Read the model definition and answer for the solid it produces. Units are mm, in the model's axes. Coordinates: 2 decimals unless noted, no trailing zeros. Write each loop counter-clockwise with the first axis right and the second up, starting at its lowest first coordinate (ties: lowest second). Pieces come first, ordered by that corner, then holes. Notation, with made-up numbers: (-23, 60.25) - (-10, 60.25) arc R23 ccw to (-10, 97.25) - close; hole circle Ø4 at (71, 35.5). An arc over 180 degrees is marked (long way). Use a Markdown table: item, result.
from build123d import *

# Parameters (mm, degrees)
ESBO_O1_W                = 45
ESBO_O1_H                = 27
RESSALTO_EXTRUS_O1_DEPTH = 1.7
RESSALTO_EXTRUS_O2_DEPTH = 1
ESBO_O3_R                = 1
CORTE_EXTRUS_O1_DEPTH    = 2.7


with BuildPart() as part:
    # Esboço1 → Ressalto-extrusão1 (new body)
    with BuildSketch(Plane(origin=(0, 0, 0), x_dir=(1, 0, 0), z_dir=(0, 1, 0))):
        with Locations((22.5, 13.5)):
            Rectangle(ESBO_O1_W, ESBO_O1_H)
    extrude(amount=RESSALTO_EXTRUS_O1_DEPTH)

    # Esboço2 → Ressalto-extrusão2 (add)
    with BuildSketch(Plane.XZ):
        Polygon((3, -22.5), (5, -24.5), (40, -24.5), (42, -22.5), (42, -4.5), (40, -2.5), (5, -2.5), (3, -4.5), align=None)
    extrude(amount=RESSALTO_EXTRUS_O2_DEPTH)

    # Esboço3 → Corte-extrusão1 (cut, through all)
    with BuildSketch(Plane.XZ):
        with Locations((2, -25)):
            Circle(ESBO_O3_R)
        with Locations((43, -25)):
            Circle(ESBO_O3_R)
        with Locations((43, -2)):
            Circle(ESBO_O3_R)
        with Locations((2, -2)):
            Circle(ESBO_O3_R)
    extrude(amount=-CORTE_EXTRUS_O1_DEPTH, mode=Mode.SUBTRACT)


solid = part.part
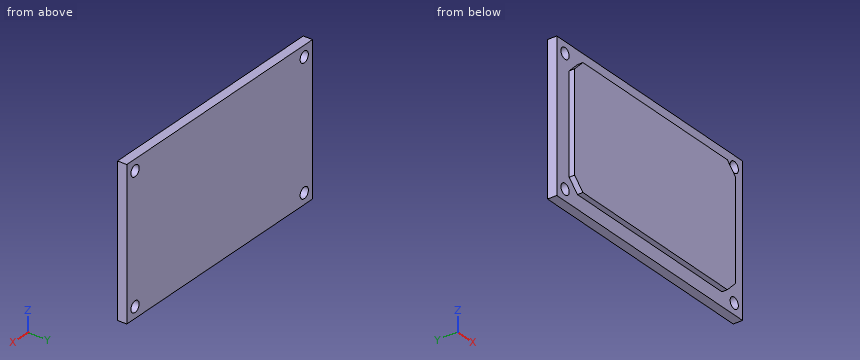
(1) A cutting plane is placed at A-A, the plane z = -25. Write down the section's boundary in (x, y), and give its area (3 significant figures).
Report:
| item | result |
|---|---|
| outline | (0, 0) - (1, 0) - (1, 1.7) - (0, 1.7) - close; (3, 0) - (42, 0) - (42, 1.7) - (3, 1.7) - close; (44, 0) - (45, 0) - (45, 1.7) - (44, 1.7) - close |
| area | 69.7 mm² |
(2) A cutting plane is placed at C-C, the plane z = -3.75. Write down the section's boundary in (x, y), and give its area (3 significant figures).
Report:
| item | result |
|---|---|
| outline | (0, 0) - (3.75, 0) - (3.75, -1) - (41.25, -1) - (41.25, 0) - (45, 0) - (45, 1.7) - (0, 1.7) - close |
| area | 114 mm² |
(3) Each of these flat-tipped pins is pushed along its axis until it touches: P1, Ø1.2, axis at x = 43, z = -25, coming from the +Y side; P2, Ø0.5, axis at x = 28, y = -0.5, coming from the +Z side; P3, Ø1.5, axis at x = 22, y = 0.5, coming from the +Z side; P4, Ø2.5, axis at x = 2, z = -25, coming from the -Y side. Where does it stop, or does it pass through?
Report:
| item | result |
|---|---|
| P1 | passes through |
| P2 | stops at z = -2.5 |
| P3 | stops at z = 0 |
| P4 | stops at y = 0 |
(4) A cutting plane is placed at D-D, the plane x = 16.5. Write down the section's boundary in (y, z), and give its area (3 significant figures).
Report:
| item | result |
|---|---|
| outline | (-1, -24.5) - (0, -24.5) - (0, -27) - (1.7, -27) - (1.7, 0) - (0, 0) - (0, -2.5) - (-1, -2.5) - close |
| area | 67.9 mm² |
(5) A cutting plane is placed at B-B, the plane x = 43. Write down the section's boundary in (y, z), and give its area (3 significant figures).
Report:
| item | result |
|---|---|
| outline | (0, -27) - (1.7, -27) - (1.7, -26) - (0, -26) - close; (0, -24) - (1.7, -24) - (1.7, -3) - (0, -3) - close; (0, -1) - (1.7, -1) - (1.7, 0) - (0, 0) - close |
| area | 39.1 mm² |
(6) Straight lines are drawn through the part: L1, parallel to Z at x = 2, y = 1; L2, parallel to Y at x = 31, z = -1.5; L3, parallel to X at y = -0.2, z = -3.25. For each, find the intervals that lie inside material, in ascending order.
Report:
| item | result |
|---|---|
| L1 | z = -27 to -26, -24 to -3, -1 to 0 |
| L2 | y = 0 to 1.7 |
| L3 | x = 4.25 to 40.75 |
